Model file for the job. Use its own axes, mm. A direction names the side the tool comes from. Round coordinates to 2 decimals unless told otherwise and drop trailing zeros. Loops run counter-clockwise (first coordinate to the right, second up) from the corner with the lowest first, then second, coordinate; pieces in that order, holes last. Notation, with made-up numbers: M -5.75,74.5 L 2.25,74.5 A28 cw 2.25,110.5 Z; hole C 79,81.25 d2. An arc over 180 degrees is marked long. Use a Markdown table: item, result. Add a question column.
Q1. Cut at A-A (y = 0.3). Give the cut face in (x, z).
Q2. Cut at C-C (x = 0). Give the cut face in (y, z), plus the area to 3 significant figures.
Q3. Pin check, flat tips, straight feed: pin 1 (5 mm diameter, centred on x = -13, z = 12, fed in from -Y); pin 2 (2.5 mm diameter, centred on x = -17.4, y = -17.1, fed in from -Z). Stop position of each tip, or through.
Q4. Probe line 1 (Y direction, x = -17.4, z = 0.75); line 2 (X direction, y = 0, z = 16.5); line 3 (Y direction, x = -13, z = 16). List the from-to ranges inside material, lowest first. Write a range as from..to.
Q5. Cut at D-D (y = 17.7). Give the cut face in (x, z), plus the area to 3 significant figures.
Q6. Cut at B-B (z = 10). Give the cut face in (x, y).
Q7. Mould opens along Y. For faces 1 (the face through (20.4, -1, 10)), 2 (the face through (17, 18, 3)), 3 (the face through (0, 20.1, 10)) say: +Y half, -Y half, draft (parallel to the pull), parting line (faces both ways), or undercut.
Q8. Tool access for faces 4 (the face through (-17, 18, 3)), 5 (the face through (-4.9, -23.2, 12.5)), 6 (the face through (-20.4, -1, 10)): list every direction of +Z, -Z, +X, -X, +Y, -Y with a clear straight run to the whole face (end or side of a thin tool).
from build123d import *

# Parameters (mm, degrees)
SKETCH2_W           = 40.8
SKETCH2_H           = 40.8
SKETCH2_R           = 1.3
SKETCH2_R_2         = 5
BOSS_EXTRUDE1_DEPTH = 20
SKETCH3_R           = 2.5
BOSS_EXTRUDE2_DEPTH = 5
SKETCH9_R           = 1.5
CUT_EXTRUDE6_DEPTH  = 3


with BuildPart() as part:
    # Sketch2 → Boss-Extrude1 (new body)
    # profile 1 of 5: a face of its own
    with BuildSketch(Plane.XY):
        with Locations((0, -0.3)):
            Rectangle(SKETCH2_W, SKETCH2_H)
        with Locations((-17.4, 17.7)):
            Circle(SKETCH2_R, mode=Mode.SUBTRACT)
        with Locations((0, 0.3)):
            Circle(SKETCH2_R_2, mode=Mode.SUBTRACT)
        with Locations((17.4, 17.7)):
            Circle(SKETCH2_R, mode=Mode.SUBTRACT)
        with Locations((17.4, -17.1)):
            Circle(SKETCH2_R, mode=Mode.SUBTRACT)
        with Locations((-17.4, -17.1)):
            Circle(SKETCH2_R, mode=Mode.SUBTRACT)
    # profile 2 of 5: a face of its own
    with BuildSketch(Plane.XY):
        with Locations((17.4, 17.7)):
            Circle(SKETCH2_R)
    # profile 3 of 5: a face of its own
    with BuildSketch(Plane.XY):
        with Locations((-17.4, -17.1)):
            Circle(SKETCH2_R)
    # profile 4 of 5: a face of its own
    with BuildSketch(Plane.XY):
        with Locations((-17.4, 17.7)):
            Circle(SKETCH2_R)
    # profile 5 of 5: a face of its own
    with BuildSketch(Plane.XY):
        with Locations((17.4, -17.1)):
            Circle(SKETCH2_R)
    extrude(amount=BOSS_EXTRUDE1_DEPTH)

    # Sketch3 → Boss-Extrude2 (add)
    with BuildSketch(Plane.XZ.offset(20.7)):
        with Locations(Location((5, 10, 0), (0, 0, 270))):
            Circle(SKETCH3_R)
        with Locations(Location((-5, 10, 0), (0, 0, 270))):
            Circle(SKETCH3_R)
    extrude(amount=BOSS_EXTRUDE2_DEPTH)

    # Sketch9 → Cut-Extrude6 (cut)
    with BuildSketch(Plane(origin=(0, 0, 0), x_dir=(-1, 0, 0), z_dir=(0, 0, -1))):
        with Locations((-17.4, 17.7)):
            Circle(SKETCH9_R)
        with Locations((17.4, 17.7)):
            Circle(SKETCH9_R)
        with Locations((17.4, -17.1)):
            Circle(SKETCH9_R)
        with Locations((-17.4, -17.1)):
            Circle(SKETCH9_R)
    extrude(amount=-CUT_EXTRUDE6_DEPTH, mode=Mode.SUBTRACT)


solid = part.part
Checked values:
| question | item | result |
|---|---|---|
| 1 | outline | M -20.4,0 L -5,0 L -5,20 L -20.4,20 Z; M 5,0 L 20.4,0 L 20.4,20 L 5,20 Z |
| 2 | outline | M -20.7,0 L -4.7,0 L -4.7,20 L -20.7,20 Z; M 5.3,0 L 20.1,0 L 20.1,20 L 5.3,20 Z |
| 2 | area | 616 mm^2 |
| 3 | pin 1 | stops at y = -20.7 |
| 3 | pin 2 | stops at z = 3 |
| 4 | line 1 | y = -20.7..-18.6, -15.6..16.2, 19.2..20.1 |
| 4 | line 2 | x = -20.4..-4.99, 4.99..20.4 |
| 4 | line 3 | y = -20.7..20.1 |
| 5 | outline | M -20.4,0 L -18.9,0 L -18.9,3 L -15.9,3 L -15.9,0 L 15.9,0 L 15.9,3 L 18.9,3 L 18.9,0 L 20.4,0 L 20.4,20 L -20.4,20 Z |
| 5 | area | 798 mm^2 |
| 6 | outline | M -20.4,-20.7 L -7.5,-20.7 L -7.5,-25.7 L -2.5,-25.7 L -2.5,-20.7 L 2.5,-20.7 L 2.5,-25.7 L 7.5,-25.7 L 7.5,-20.7 L 20.4,-20.7 L 20.4,20.1 L -20.4,20.1 Z; hole C 0,0.3 d10 |
| 7 | face 1 | draft |
| 7 | face 2 | undercut |
| 7 | face 3 | +Y half |
| 8 | face 4 | -Z |
| 8 | face 5 | -Y |
| 8 | face 6 | +Z, -Z, -X, +Y, -Y |
